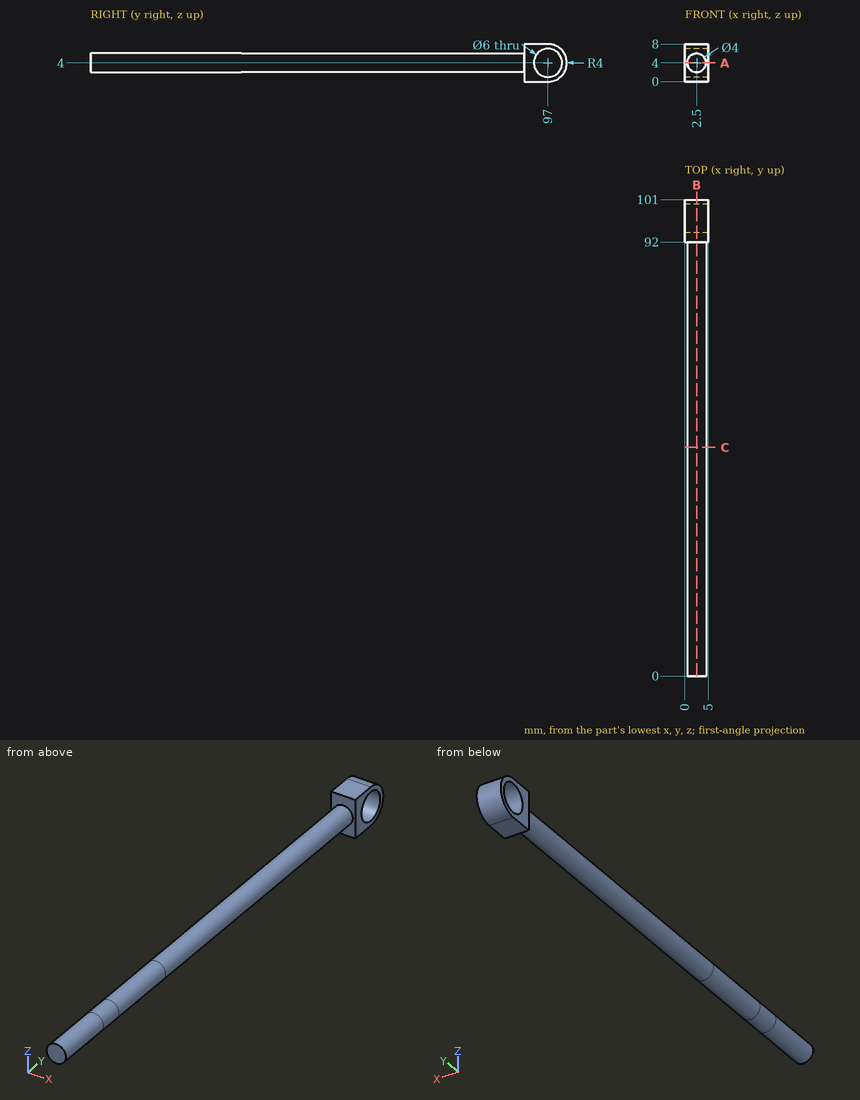
Part print with two shaded views. Sizes in mm from the minimum x, y, z corner. Give positions to 0.01 mm unless a question says otherwise; leave off trailing zeros. Write each loop counter-clockwise with the first axis right and the second up, starting at its lowest first coordinate (ties: lowest second). Pieces come first, ordered by that corner, then holes.
1) Cut at B-B on x = 2.5. Write the cut outline in (y, z), then the cut area to 3 significant figures.
Resolved:
outline: (0, 2) - (92, 2) - (92, 0) - (97, 0) arc R4 ccw to (97, 8) - (92, 8) - (92, 6) - (0, 6) - close; hole circle Ø6 at (97, 4)
area: 405 mm2
2) Pin check, flat tips, straight feed: pin 1 (1.5 mm diameter, centred on y = 68, z = 6.5, fed in from +X); pin 2 (3 mm diameter, centred on x = 4, y = 68.5, fed in from +Z). Stop position of each tip, or through.
Resolved:
pin 1: stops at x = 3.47
pin 2: stops at z = 6
3) Cut at C-C on y = 48.5. Write the cut outline in (x, z).
Resolved:
outline: circle Ø4 at (2.5, 4)
4) Cut at A-A on z = 4. Write the cut outline in (x, y).
Resolved:
outline: (0, 92) - (0.5, 92) - (0.5, 0) - (4.5, 0) - (4.5, 92) - (5, 92) - (5, 94) - (0, 94) - close; (0, 100) - (5, 100) - (5, 101) - (0, 101) - close
5) Probe L1, parallel to Y at x = 1.9, z = 4; L2, parallel to X at y = 13.5, z = 4.25; L3, parallel to Y at x = 3.6, z = 2.5. List the from-to ranges inside material, lowest first.
Resolved:
L1: y = 0 to 94, 100 to 101
L2: x = 0.52 to 4.48
L3: y = 0 to 94.4, 99.6 to 100.71
